Verification items for the finished model (mm, model axes). Face numbers are marked on the shaded views. A direction names the side the tool comes from. Coordinates: 2 decimals unless noted, no trailing zeros. Order: outer loops, then holes, each group sorted by start corner. A loop starts at its lowest first (then second) coordinate and runs counter-clockwise, first axis right, second up. Notation, with made-up numbers: M -5,-9.5 L 10,-9.5 A8 ccw 10,1.5 Z; hole C -19.5,6 d9. An arc over 180 degrees is marked long. Return JSON: item names as keys, results as strings.
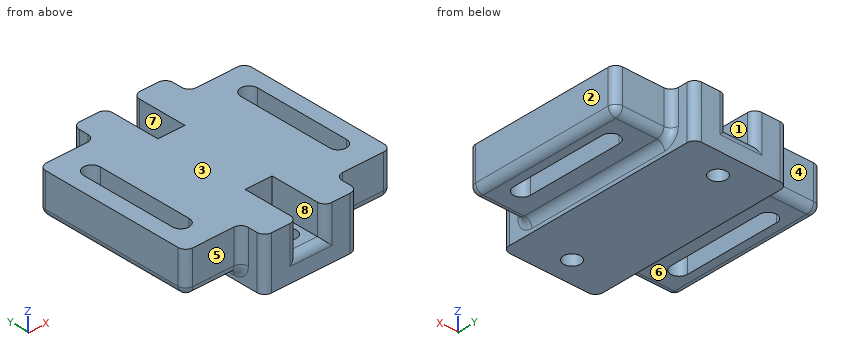
```python
from build123d import *

# Parameters (mm, degrees)
BOSS_EXTRUDE1_DEPTH      = 55
M4_CLEARANCE_HOLE1_D     = 4.5
M4_CLEARANCE_SLOT1_DEPTH = 11
SKETCH6_W                = 7.2
SKETCH6_H                = 8
CUT_EXTRUDE1_DEPTH       = 15
SKETCH7_W                = 15
SKETCH7_H                = 6.5
CUT_EXTRUDE3_DEPTH       = 79.555712714
MIRROR3_COPY_1_SKETCH_W  = 15
MIRROR3_COPY_1_SKETCH_H  = 6.5
MIRROR3_COPY_1_DEPTH     = 79.555712714
FILLET1_R                = 2


# Read off the part's stored shape, not the designer's step: M4 Clearance Slot1
with BuildPart() as part:
    # Sketch1 → Boss-Extrude1 (new body)
    with BuildSketch(Plane(origin=(0, 0, 0), x_dir=(1, 0, 0), z_dir=(0, 1, 0))):
        Polygon((0, 0), (15, 0), (15, 3), (40, 3), (40, 0), (55, 0), (55, -11), (0, -11), align=None)
    extrude(amount=BOSS_EXTRUDE1_DEPTH)

    # M4 Clearance Hole1 (through all)
    with Locations(Plane(origin=(0, 0, -3), x_dir=(-1, 0, 0), z_dir=(0, 0, -1))):
        with Locations((-27.5, 48.435), (-27.5, 6.565)):
            Hole(M4_CLEARANCE_HOLE1_D / 2)

    # M4 Clearance Slot1 outline → M4 Clearance Slot1 (cut)
    with BuildSketch(Plane.XY):
        with BuildLine():
            ThreePointArc((46.25, 14.75), (48.5, 12.5), (50.75, 14.75))
            Line((50.75, 14.75), (50.75, 40.25))
            ThreePointArc((50.75, 40.25), (48.5, 42.5), (46.25, 40.25))
            Line((46.25, 40.25), (46.25, 14.75))
        make_face()
        with BuildLine():
            ThreePointArc((4.25, 14.75), (6.5, 12.5), (8.75, 14.75))
            Line((8.75, 14.75), (8.75, 40.25))
            ThreePointArc((8.75, 40.25), (6.5, 42.5), (4.25, 40.25))
            Line((4.25, 40.25), (4.25, 14.75))
        make_face()
    extrude(amount=M4_CLEARANCE_SLOT1_DEPTH, mode=Mode.SUBTRACT)

    # Sketch6 → Cut-Extrude1 (cut)
    with BuildSketch(Plane(origin=(0, 55, 0), x_dir=(1, 0, 0), z_dir=(0, 1, 0))):
        with Locations((27.5, -7)):
            Rectangle(SKETCH6_W, SKETCH6_H)
    cut_extrude1 = extrude(amount=-CUT_EXTRUDE1_DEPTH, mode=Mode.SUBTRACT)

    # Mirror1: Cut-Extrude1 across plane
    add(cut_extrude1.mirror(Plane.ZX.offset(27.5)), mode=Mode.SUBTRACT)

    # Sketch7 → Cut-Extrude3 (cut, through all)
    with BuildSketch(Plane(origin=(0, 0, 0), x_dir=(-1, 0, 0), z_dir=(0, 0, -1))):
        with Locations((-7.5, 3.25)):
            Rectangle(SKETCH7_W, SKETCH7_H)
    cut_extrude3 = extrude(amount=-CUT_EXTRUDE3_DEPTH, mode=Mode.SUBTRACT)

    # Mirror2: Cut-Extrude3 across plane
    add(cut_extrude3.mirror(Plane(origin=(0, 27.5, 0), x_dir=(0, 0, 1), z_dir=(0, -1, 0))), mode=Mode.SUBTRACT)

    # Mirror3: Cut-Extrude3 across plane
    add(cut_extrude3.mirror(Plane(origin=(27.5, 0, 0), x_dir=(0, 0, 1), z_dir=(1, 0, 0))), mode=Mode.SUBTRACT)

    # Mirror3 copy 1 sketch → Mirror3 copy 1 (cut, through all)
    with BuildSketch(Plane(origin=(55, 55, 0), x_dir=(1, 0, 0), z_dir=(0, 0, -1))):
        with Locations((-7.5, 3.25)):
            Rectangle(MIRROR3_COPY_1_SKETCH_W, MIRROR3_COPY_1_SKETCH_H)
    extrude(amount=-MIRROR3_COPY_1_DEPTH, mode=Mode.SUBTRACT)

    # Fillet1
    fillet1_edges = [part.edges().sort_by_distance(p)[0] for p in [
        (7.5, 6.5, 0),
        (15, 27.5, 0),
        (0, 27.5, 0),
        (15, 48.5, 5.5),
        (7.5, 48.5, 0),
        (0, 48.5, 5.5),
        (40, 27.5, 0),
        (55, 27.5, 0),
        (40, 48.5, 5.5),
        (55, 48.5, 5.5),
        (47.5, 48.5, 0),
        (40, 6.5, 5.5),
        (47.5, 6.5, 0),
        (55, 6.5, 5.5),
        (40, 55, 4),
        (15, 55, 4),
        (23.9, 55, 7),
        (31.1, 55, 7),
        (27.5, 55, 3),
        (27.5, 0, 3),
        (23.9, 0, 7),
        (31.1, 0, 7),
        (15, 0, 4),
        (40, 0, 4),
        (15, 6.5, 5.5),
        (0, 6.5, 5.5),
    ]]
    fillet(fillet1_edges, radius=FILLET1_R)


solid = part.part
```
Q1. Tool access check on the marked faces 4, 5, 6, 7 and 8. Record the directions out of +Z, -Z, +X, -X, +Y, -Y that give a thin tool (end or side, any length) a straight path to the whole face; none if there is none.
Values:
{"face 4": "+Z, -Z, -X, +Y", "face 5": "+Z, -Z, -X, -Y", "face 6": "-Z, -X, +Y, -Y", "face 7": "+Z, +Y", "face 8": "+Z, -Y"}
Q2. Draft check along X on the marked faces 1, 2 and 3. Enter one of: pulls with the +X half, pulls with the -X half, needs draft (parallel to the pull), parting line crosses it, or undercut.
Values:
{"face 1": "undercut", "face 2": "pulls with the +X half", "face 3": "needs draft"}
Q3. Material ranges on line 1 along Y through (x, z) = (27.5, -0.75) (3 decimals); line 2 along X through (y, z) = (23, 9.25); line 3 along X through (y, z) = (45, 9), recorded low to high.
Values:
{"line 1": "0 to 4.315, 8.815 to 46.185, 50.685 to 55", "line 2": "0 to 4.25, 8.75 to 46.25, 50.75 to 55", "line 3": "0 to 23.9, 31.1 to 55"}
Q4. Cross-section at C-C, the plane x = 48.5. Record the boundary of the cut face in (y, z), and give its area (3 significant figures).
Values:
{"outline": "M 6.5,2 A2 ccw 8.5,0 L 12.5,0 L 12.5,11 L 6.5,11 Z; M 42.5,0 L 46.5,0 A2 ccw 48.5,2 L 48.5,11 L 42.5,11 Z", "area": "130 mm^2"}
Q5. Go/stop test with flat-tipped pins: pin 1 (1 mm diameter, centred on x = 45, z = 4, fed in from +Y); pin 2 (1.5 mm diameter, centred on x = 45, z = 3, fed in from -Y); pin 3 (2.5 mm diameter, centred on y = 5.5, z = 9, fed in from +X). Record where each tip stops, or that it passes through.
Values:
{"pin 1": "y = 48.5", "pin 2": "y = 6.5", "pin 3": "x = 53.97"}
Q6. Cross-section at D-D, the plane z = 6.5. State how many separate pieces and enclosed holes the cut face has, and give its area (3 significant figures).
Values:
{"separate pieces": "1", "enclosed holes": "2", "area": "2,150 mm^2"}
Q7. Cross-section at B-B, the plane x = 27.5. Record the boundary of the cut face in (y, z) (3 decimals), and give its area (3 significant figures).
Values:
{"outline": "M 0,-3 L 4.315,-3 L 4.315,3 L 2,3 A2 ccw 0,1 Z; M 8.815,-3 L 46.185,-3 L 46.185,3 L 40,3 L 40,11 L 15,11 L 15,3 L 8.815,3 Z; M 50.685,-3 L 55,-3 L 55,1 A2 ccw 53,3 L 50.685,3 Z", "area": "474 mm^2"}
Q8. Cross-section at A-A, the plane y = 28. Record the boundary of the cut face in (x, z).
Values:
{"outline": "M 0,2 A2 ccw 2,0 L 4.25,0 L 4.25,11 L 0,11 Z; M 8.75,0 L 13,0 A2 cw 15,-2 L 15,-3 L 40,-3 L 40,-2 A2 cw 42,0 L 46.25,0 L 46.25,11 L 8.75,11 Z; M 50.75,0 L 53,0 A2 ccw 55,2 L 55,11 L 50.75,11 Z"}
